Geometry check sheet. Reference: the model listing, model coordinates, mm. Give positions to 0.01 mm unless a question says otherwise; leave off trailing zeros. Loops run counter-clockwise (first coordinate to the right, second up) from the corner with the lowest first, then second, coordinate; pieces in that order, holes last. Notation, with made-up numbers: (-36.75, 9.25) -> (-4.75, 9.25) arc R31 cw to (-4.75, 47.25) -> close; hole circle Ø10 at (-2, 77). An arc over 180 degrees is marked (long way). Answer in a Markdown table with one row per item. Add a question column.
```python
from build123d import *

# Parameters (mm, degrees)
F1_DEPTH = 5.0546
F2_D     = 1.27
F4_DEPTH = 25.4


# Not quite as in the source:
# - a feature names something its author has since deleted; it is built from what else it names


with BuildPart() as f1:
    # F0 (on Front) → F1 (new body)
    with BuildSketch(Plane.XZ):
        Polygon((-45.5380498264, 42.9229369958), (-51.539901644, 42.8869388998), (-45.5468128822, 42.675064641), align=None)
        with BuildLine():
            Line((-45.5468128822, 42.675064641), (-51.539901644, 42.8869388998))
            ThreePointArc((-51.539901644, 42.8869388998), (-51.187813042, 41.162667719), (-50.1936934888, 39.710495621))
            Line((-50.1936934888, 39.710495621), (-47.0142699778, 39.6847687662))
            ThreePointArc((-47.0142699778, 39.6847687662), (-45.9490353675, 41.0264089842), (-45.474623776, 42.6725125324))
            Line((-45.474623776, 42.6725125324), (-45.5468128822, 42.675064641))
        make_face()
    extrude(amount=F1_DEPTH)

    # F2 (through all)
    with Locations(Plane(origin=(0, 0, 0), x_dir=(1, 0, 0), z_dir=(0, 1, 0))):
        with Locations((-48.6222168853, -41.1340259016)):
            Hole(F2_D / 2)

    # F3 (on face) → F4 (cut)
    with BuildSketch(Plane(origin=(0.3180170752, 0, 39.3017713856), x_dir=(0.999967264, 0, -0.0080914079), z_dir=(-0.0080914079, 0, -0.999967264))):
        Polygon((-50.5133641684, 2.0186165348), (-48.9236003704, 2.0186165348), (-47.3338365724, 2.0186165348), (-47.3338365724, 3.0329779256), (-50.5133641684, 3.0329779256), align=None)
    extrude(amount=-F4_DEPTH, mode=Mode.SUBTRACT)


solid = f1.part
```
1. Sectioned sample at D-D (x = -48.25). Enter the section's corners in (y, z).
2. Release check for a two-part mould opening along Z. For faces 1 (the face through (-48.964, -1.023, 40.599)), 2 (the face through (-49, 0, 42)), 3 (the face through (-45.96, -2.492, 41.005)) record: released by +Z, released by -Z, zero draft, split by the parting line, or undercut.
3. Sectioned sample at A-A (y = -2.95). Enter the section's corners in (x, z).
4. Material ranges on L1, parallel to Y at x = -47.5, z = 42.4; L2, parallel to X at y = -2.9, z = 41.25; L3, parallel to X at y = -2.15, z = 40.8, recorded low to high. Write a range as from..to.
5. Sectioned sample at B-B (x = -47.5). Enter the section's corners in (y, z).
6. Sectioned sample at C-C (z = 40.8). Enter the section's corners in (x, y), plus the area to 3 significant figures.
7. Gauge pin test, flat ends, axial feed: pin 1 Ø1 at (x, z) = (-48.62, 41.13) entering from -Y; pin 2 Ø1 at (y, z) = (-3.5, 40) entering from +X. Record the tip position at first contact, or that the pin passes through.
Response:
| question | item | result |
|---|---|---|
| 1 | outline | (-5.05, 39.69) -> (-3.03, 39.69) -> (-3.03, 40.62) -> (-5.05, 40.62) -> close; (-5.05, 41.65) -> (-3.03, 41.65) -> (-3.03, 42.91) -> (-5.05, 42.91) -> close; (-2.02, 39.69) -> (0, 39.69) -> (0, 40.62) -> (-2.02, 40.62) -> close; (-2.02, 41.65) -> (0, 41.65) -> (0, 42.91) -> (-2.02, 42.91) -> close |
| 2 | face 1 | undercut |
| 2 | face 2 | zero draft |
| 2 | face 3 | released by -Z |
| 3 | outline | (-51.54, 42.89) arc R4.44 ccw to (-50.19, 39.71) -> (-50.17, 42.9) -> close; (-47.01, 39.68) arc R4.42 ccw to (-45.47, 42.67) -> (-45.55, 42.68) -> (-45.54, 42.92) -> (-46.99, 42.91) -> close |
| 4 | L1 | y = -5.05..-3.03, -2.02..0 |
| 4 | L2 | x = -51.22..-50.18, -47..-45.84 |
| 4 | L3 | x = -51.01..-50.18, -47.01..-46.07 |
| 5 | outline | (-5.05, 39.69) -> (-3.03, 39.69) -> (-3.03, 42.91) -> (-5.05, 42.91) -> close; (-2.02, 39.69) -> (0, 39.69) -> (0, 42.91) -> (-2.02, 42.91) -> close |
| 6 | outline | (-51.01, -5.05) -> (-49.16, -5.05) -> (-49.16, -3.03) -> (-50.18, -3.03) -> (-50.18, -2.02) -> (-49.16, -2.02) -> (-49.16, 0) -> (-51.01, 0) -> close; (-48.08, -5.05) -> (-46.07, -5.05) -> (-46.07, 0) -> (-48.08, 0) -> (-48.08, -2.02) -> (-47.01, -2.02) -> (-47.01, -3.03) -> (-48.08, -3.03) -> close |
| 6 | area | 17.4 mm2 |
| 7 | pin 1 | passes through |
| 7 | pin 2 | stops at x = -46.27 |
